Print and shaded views of the part. All mm, measured from the part's lowest x, y and z. A direction names the side the tool comes from. Give positions to 0.01 mm unless a question says otherwise; leave off trailing zeros. Order: outer loops, then holes, each group sorted by start corner. A loop starts at its lowest first (then second) coordinate and runs counter-clockwise, first axis right, second up. Notation, with made-up numbers: (22, -0.5) -> (49, -0.5) arc R9 ccw to (49, 7.5) -> close; hole circle Ø3 at (21, 83). An arc over 180 degrees is marked (long way). One line per question, with ' | ' between items. Start each with the question number.
(1) Cut at C-C (y = 5). Give the cut face in (x, z).
(2) Which spindle directions (+Z, -Z, +X, -X, +Y, -Y) get a long thin tool onto all of the face, cutting with end or side? Do the marked faces 1, 2 and 3. Say none if no direction does.
(3) Cut at A-A (x = 3). Give the cut face in (y, z).
(4) Cut at D-D (z = 4.45). Give the cut face in (x, y).
(5) Pull direction X, two halves, no side cores. Call the marked faces 4, 5 and 6: +X half, -X half, draft (parallel to the pull), parting line (faces both ways), or undercut.
(6) Cut at B-B (y = 8.25). Give the cut face in (x, z), then the cut area to 3 significant figures.
(7) Pin check, flat tips, straight feed: pin 1 Ø1 at (y, z) = (5, 4.5) entering from -X; pin 2 Ø1.3 at (x, y) = (2.5, 6.5) entering from +Z; pin 3 Ø2.5 at (x, y) = (3, 8) entering from -Z; pin 4 Ø1.3 at (x, y) = (3, 6) entering from -Z. Stop position of each tip, or through.
(8) Drill centre lines: L1, parallel to Y at x = 3, z = 3.6; L2, parallel to X at y = 7.5, z = 2.3; L3, parallel to X at y = 8.5, z = 3.1. Where is each one in solid material? Low to high. Write a range as from..to.
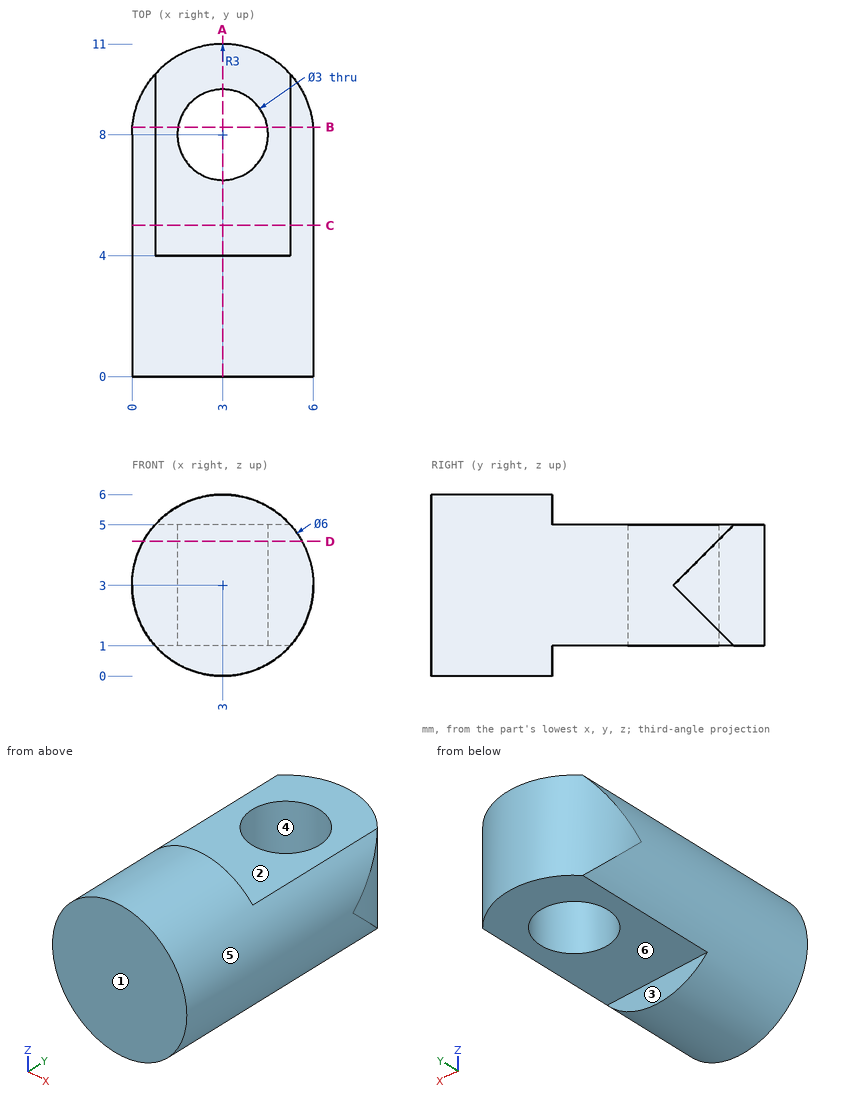
Result set:
1) outline: (0.76, 1) -> (5.24, 1) arc R3 ccw to (5.24, 5) -> (0.76, 5) arc R3 ccw to start
2) face 1: +Z, -Z, +X, -X, -Y | face 2: +Z, +X, -X, +Y | face 3: -Z, +X, -X, +Y
3) outline: (0, 0) -> (4, 0) -> (4, 1) -> (6.5, 1) -> (6.5, 5) -> (4, 5) -> (4, 6) -> (0, 6) -> close; (9.5, 1) -> (11, 1) -> (11, 5) -> (9.5, 5) -> close
4) outline: (0.37, 0) -> (5.63, 0) -> (5.63, 9.45) arc R3 ccw to (0.37, 9.45) -> close; hole circle Ø3 at (3, 8)
5) face 4: undercut | face 5: parting line | face 6: draft
6) outline: (0.01, 2.75) arc R3 ccw to (0.76, 1) -> (1.52, 1) -> (1.52, 5) -> (0.76, 5) arc R3 ccw to (0.01, 3.25) -> close; (4.48, 1) -> (5.24, 1) arc R3 ccw to (5.99, 2.75) -> (5.99, 3.25) arc R3 ccw to (5.24, 5) -> (4.48, 5) -> close | area: 10.2 mm2
7) pin 1: stops at x = 0.17 | pin 2: stops at z = 5 | pin 3: passes through | pin 4: stops at z = 1
8) L1: y = 0..6.5, 9.5..11 | L2: x = 0.08..1.59, 4.41..5.92 | L3: x = 0.04..1.59, 4.41..5.96
